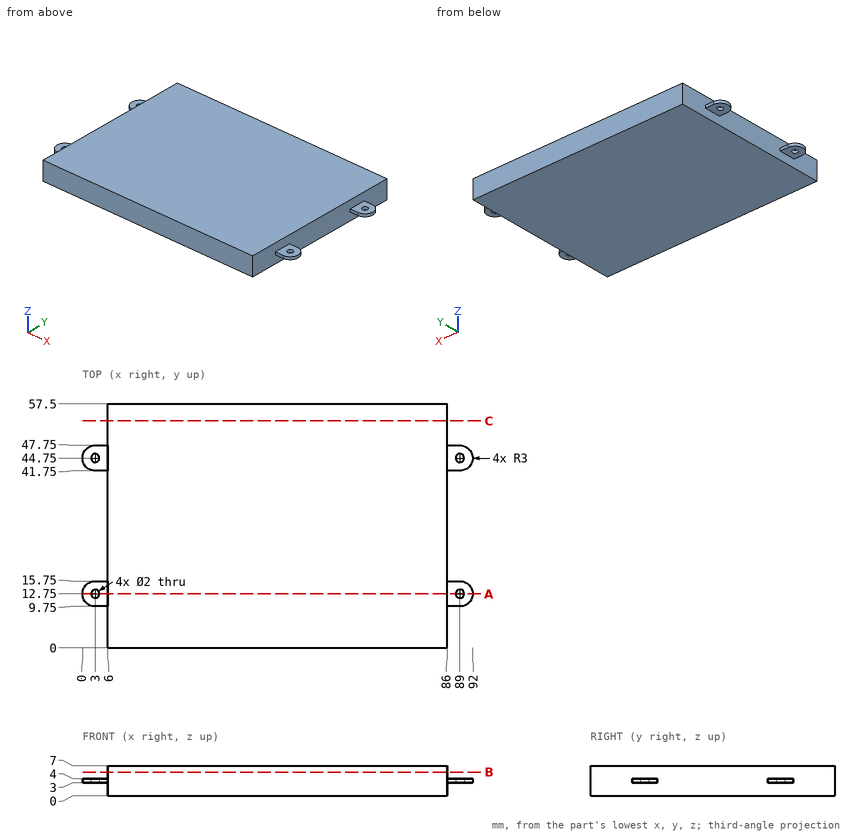
For this review, use the dimensioned drawing (mm, ordinates from the lowest corner) and the shaded views. Round coordinates to 2 decimals unless told otherwise and drop trailing zeros. Write each loop counter-clockwise with the first axis right and the second up, starting at its lowest first coordinate (ties: lowest second). Pieces come first, ordered by that corner, then holes. Notation, with made-up numbers: (26.5, -8.5) -> (70.5, -8.5) arc R24 ccw to (70.5, 26.5) -> close; hole circle Ø5 at (85.25, -39.75). An arc over 180 degrees is marked (long way). Use CSV: the item, a comma, the result in double quotes.
Q1. To check wall thickness, follow probe 1 along X at (y, z) = (44.75, 3.5); probe 2 along Y at (x, z) = (3, 3.8); probe 3 along X at (y, z) = (3, 1.5). State the ranges of each line that lie inside material, in increasing order. Write a range as [from, to].
Checks:
probe 1,"[0, 2], [4, 88], [90, 92]"
probe 2,"[9.75, 11.75], [13.75, 15.75], [41.75, 43.75], [45.75, 47.75]"
probe 3,"[6, 86]"
Q2. For pin 1 Ø1.2 at (x, y) = (3, 44.75) entering from -Z; pin 2 Ø1.8 at (x, y) = (90, 13) entering from +Z; pin 3 Ø1.1 at (x, z) = (4.5, 3.5) entering from -Y; pin 4 Ø1.8 at (x, y) = (2, 11.5) entering from -Z, all flat-tipped, find the tip position at first contact; note any pin that passes through.
Checks:
pin 1,"through"
pin 2,"z = 4"
pin 3,"y = 9.75"
pin 4,"z = 3"
Q3. Consider section A-A (y = 12.75). Give the boundary of the cut face in (x, z).
Checks:
outline,"(0, 3) -> (2, 3) -> (2, 4) -> (0, 4) -> close; (4, 3) -> (6, 3) -> (6, 0) -> (86, 0) -> (86, 3) -> (88, 3) -> (88, 4) -> (86, 4) -> (86, 7) -> (6, 7) -> (6, 4) -> (4, 4) -> close; (90, 3) -> (92, 3) -> (92, 4) -> (90, 4) -> close"
Q4. Consider section B-B (z = 5.5). Give the boundary of the cut face in (x, y), then the cut area to 3 significant figures.
Checks:
outline,"(6, 0) -> (86, 0) -> (86, 57.5) -> (6, 57.5) -> close"
area,"4,600 mm²"
Q5. Consider section C-C (y = 53.5). Give the boundary of the cut face in (x, z).
Checks:
outline,"(6, 0) -> (86, 0) -> (86, 7) -> (6, 7) -> close"
